Geometry: final body of the model. Coordinates: model frame, mm. Face numbers are marked on the shaded views. Coordinates: 2 decimals unless noted, no trailing zeros. Order: outer loops, then holes, each group sorted by start corner. A loop starts at its lowest first (then second) coordinate and runs counter-clockwise, first axis right, second up. Notation, with made-up numbers: M 70,20 L 83,20 A23 ccw 83,58 Z; hole C 83.25,-4 d7. An arc over 180 degrees is marked long. Write item = value, one per line.
from build123d import *

# Parameters (mm, degrees)
EXTRUDE_1_4_DEPTH       = 3.1
CUT_EXTRUDE2_DEPTH      = 3.1
CUT_EXTRUDE2_DEPTH_BACK = 8
SKETCH3_R               = 11.25
SKETCH2_R               = 1.3
M3_DRILL_DEPTH          = 6.2
SKETCH4_R               = 1.7
M4_DRILL_DEPTH          = 8
SKETCH5_R               = 1.7
M4_DRILL2_DEPTH         = 8
SKETCH6_R               = 2.2
M4_THROUGH_DEPTH        = 6.2


with BuildPart() as part:
    # Sketch1 → 1/4 (new, symmetric)
    with BuildSketch(Plane.XY):
        Polygon((-20, 45), (20, 45), (30, 10), (30, -45), (-30, -45), (-30, 10), align=None)
    extrude(amount=EXTRUDE_1_4_DEPTH, both=True)

    # Sketch3 → Cut-Extrude2 (cut, two sides: drawn at the far end of the back side and taken through both)
    with BuildSketch(Plane.XY.offset(-CUT_EXTRUDE2_DEPTH_BACK)):
        Circle(SKETCH3_R)
    extrude(amount=CUT_EXTRUDE2_DEPTH + CUT_EXTRUDE2_DEPTH_BACK, mode=Mode.SUBTRACT)

    # Sketch2 → M3_DRILL (cut)
    with BuildSketch(Plane.XY.offset(3.1)):
        with Locations((-9.899494937, 9.899494937)):
            Circle(SKETCH2_R)
        with Locations((9.899494937, 9.899494937)):
            Circle(SKETCH2_R)
        with Locations((9.899494937, -9.899494937)):
            Circle(SKETCH2_R)
        with Locations((-9.899494937, -9.899494937)):
            Circle(SKETCH2_R)
    extrude(amount=-M3_DRILL_DEPTH, mode=Mode.SUBTRACT)

    # Sketch4 → M4_DRILL (cut)
    with BuildSketch(Plane(origin=(0, 45, 0), x_dir=(1, 0, 0), z_dir=(0, 1, 0))):
        with Locations(Location((-12, 0, 0), (0, 0, 180))):
            Circle(SKETCH4_R)
        with Locations((12, 0)):
            Circle(SKETCH4_R)
    extrude(amount=-M4_DRILL_DEPTH, mode=Mode.SUBTRACT)

    # Sketch5 → M4_DRILL2 (cut)
    with BuildSketch(Plane(origin=(0, -45, 0), x_dir=(-1, 0, 0), z_dir=(0, -1, 0))):
        with Locations(Location((-20, 0, 0), (0, 0, 180))):
            Circle(SKETCH5_R)
        with Locations((20, 0)):
            Circle(SKETCH5_R)
        with Locations(Location((0, 0, 0), (0, 0, 180))):
            Circle(SKETCH5_R)
    extrude(amount=-M4_DRILL2_DEPTH, mode=Mode.SUBTRACT)

    # Sketch6 → M4_through (cut)
    with BuildSketch(Plane.XY.offset(3.1)):
        with Locations((-25.2375, -31)):
            Circle(SKETCH6_R)
        with Locations((25.2375, -31)):
            Circle(SKETCH6_R)
        with Locations((-15.2375, 31)):
            Circle(SKETCH6_R)
        with Locations((15.2375, 31)):
            Circle(SKETCH6_R)
    extrude(amount=-M4_THROUGH_DEPTH, mode=Mode.SUBTRACT)


solid = part.part
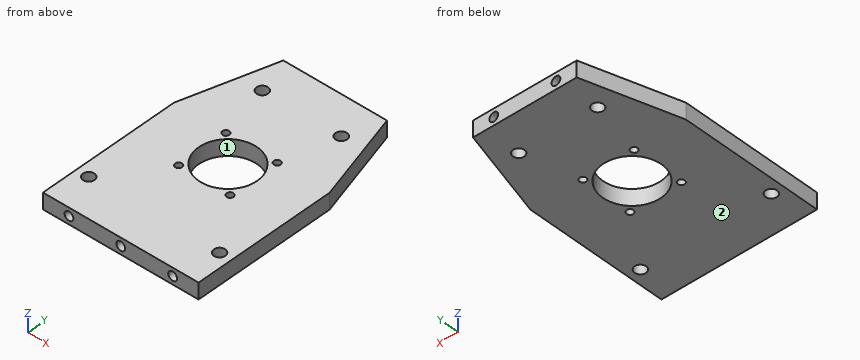
1) Section C-C, the plane x = -5. Return loops of the section in (y, z).
Numbers:
outline = M -45,-3.1 L -10.08,-3.1 L -10.08,3.1 L -45,3.1 Z; M 10.08,-3.1 L 45,-3.1 L 45,3.1 L 10.08,3.1 Z
2) Line query: L1, parallel to Z at x = 12, y = 41; L2, parallel to X at y = 10, z = -1; L3, parallel to X at y = -29.5, z = 2. Output: solid intervals per line, ascending.
Numbers:
L1 = -3.1 to -1.7, 1.7 to 3.1
L2 = -30 to -11.2, -8.6 to -5.15, 5.15 to 8.6, 11.2 to 30
L3 = -30 to -26.85, -23.63 to 23.63, 26.85 to 30
3) Section D-D, the plane z = 0. Give the number of separate pieces and of enclosed holes in the cut face, and give its area (3 significant figures).
Numbers:
separate_pieces = 1
enclosed_holes = 9
area = 4,430 mm²
4) Pin query (flat end, axial travel): pin 1 (2.5 mm diameter, centred on x = 9.9, y = -9.9, fed in from -Z); pin 2 (3 mm diameter, centred on x = 0, z = 0, fed in from -Y); pin 3 (1.7 mm diameter, centred on x = -12.5, z = 0.5, fed in from +Y). Return the tip coordinate at first contact, or that it passes through.
Numbers:
pin_1 = through
pin_2 = -37
pin_3 = 37
5) Mould query, pull axis X, two halves, no side actions, for the marked faces 1 and 2. Classes: pulls with the +X half, pulls with the -X half, needs draft (parallel to the pull), parting line crosses it, or undercut.
Numbers:
face_1 = undercut
face_2 = needs draft
6) Section B-B, the plane y = 0. Return loops of the section in (x, z), and give its area (4 significant figures).
Numbers:
outline = M -30,-3.1 L -11.25,-3.1 L -11.25,3.1 L -30,3.1 Z; M 11.25,-3.1 L 30,-3.1 L 30,3.1 L 11.25,3.1 Z
area = 232.5 mm²
7) Section A-A, the plane y = 31. Return loops of the section in (x, z).
Numbers:
outline = M -24,-3.1 L -17.44,-3.1 L -17.44,3.1 L -24,3.1 Z; M -13.04,-3.1 L 13.04,-3.1 L 13.04,3.1 L -13.04,3.1 Z; M 17.44,-3.1 L 24,-3.1 L 24,3.1 L 17.44,3.1 Z
